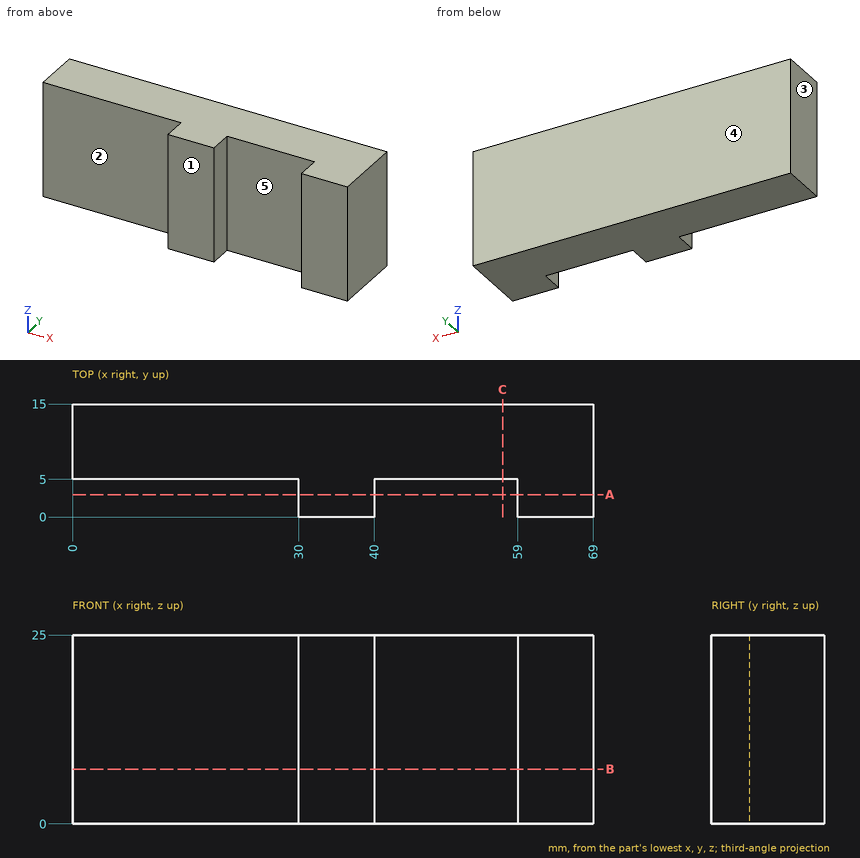
Source: three-view drawing plus pictorial views. Frame: mm from the lowest corner of the part. A direction names the side the tool comes from. Give positions to 0.01 mm unless a question says otherwise; leave off trailing zeros. Order: outer loops, then holes, each group sorted by start corner. A loop starts at its lowest first (then second) coordinate and runs counter-clockwise, first axis right, second up. Notation, with made-up numbers: M 86,19 L 144,19 A13 ccw 144,26 Z; hole C 85,14 d7. An arc over 180 degrees is marked long. One line per question, with ' | ' between items.
1) Section B-B on z = 7.25. Output: boundary loops of the cut face in (x, y).
Filled in:
outline: M 0,5 L 30,5 L 30,0 L 40,0 L 40,5 L 59,5 L 59,0 L 69,0 L 69,15 L 0,15 Z
2) Contact query for flat-ended pins moving along their axis: P1, Ø5, axis at x = 26.5, z = 17, coming from the -Y side; P2, Ø1.5, axis at y = 3, z = 13, coming from the -X side. Output: stop coordinate, or through.
Filled in:
P1: stops at y = 5 | P2: stops at x = 30
3) Section A-A on y = 3. Output: boundary loops of the cut face in (x, z).
Filled in:
outline: M 30,0 L 40,0 L 40,25 L 30,25 Z; M 59,0 L 69,0 L 69,25 L 59,25 Z
4) Draft query along X for the marked faces 3, 4 and 5. Return one class per face: pulls with the +X half, pulls with the -X half, needs draft (parallel to the pull), parting line crosses it, or undercut.
Filled in:
face 3: pulls with the -X half | face 4: needs draft | face 5: undercut
5) Ray query, L1, parallel to Y at x = 53, z = 2.75. Return the intervals inside material, ascending.
Filled in:
L1: y = 5 to 15
6) Section C-C on x = 57. Output: boundary loops of the cut face in (y, z).
Filled in:
outline: M 5,0 L 15,0 L 15,25 L 5,25 Z
7) Access query for the marked faces 1 and 2. Directions: +Z, -Z, +X, -X, +Y, -Y. A direction counts if a zero-diameter tool reaches every point of the face in a straight line with its end or side. Return the directions, or none.
Filled in:
face 1: +Z, -Z, +X, -X, -Y | face 2: +Z, -Z, -X, -Y
